Geometry check sheet. Reference: the model listing, model coordinates, mm. Face numbers are marked on the shaded views. A direction names the side the tool comes from. Round coordinates to 2 decimals unless told otherwise and drop trailing zeros. Write each loop counter-clockwise with the first axis right and the second up, starting at its lowest first coordinate (ties: lowest second). Pieces come first, ordered by that corner, then holes. Notation, with made-up numbers: (36.5, 31) - (69.5, 31) arc R22 ccw to (69.5, 39) - close; hole circle Ø2 at (43.25, -14.75). An arc over 180 degrees is marked (long way). Return JSON: item names as keys, results as strings. Group by question number.
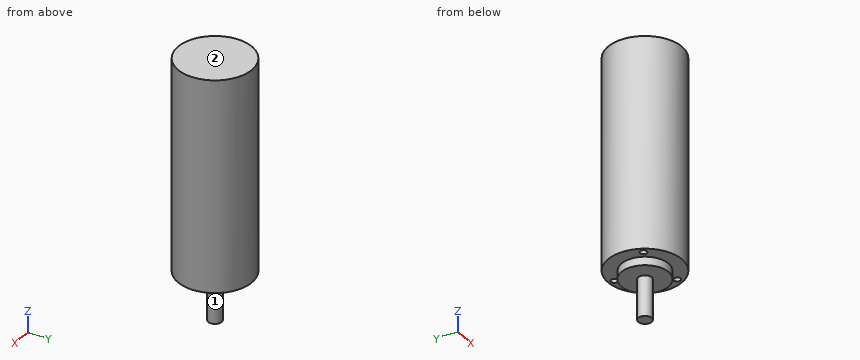
from build123d import *

# Parameters (mm, degrees)
SKETCH2_R          = 1
CUT_EXTRUDE1_DEPTH = 3


with BuildPart() as part:
    # Sketch1 → Revolve1 (revolve)
    with BuildSketch(Plane(origin=(0, 0, 0), x_dir=(1, 0, 0), z_dir=(0, 1, 0))):
        Polygon((0, 0), (11, 0), (11, 62.8), (7, 62.8), (7, 65.3), (2, 65.3), (2, 77.3), (0, 77.3), align=None)
    revolve(axis=Axis((0, 0, 0), (0, 0, -1)))

    # Sketch2 → Cut-Extrude1 (cut)
    with BuildSketch(Plane(origin=(0, 0, -62.8), x_dir=(-1, 0, 0), z_dir=(0, 0, -1))):
        with Locations((-8, -4.618802154)):
            Circle(SKETCH2_R)
        with Locations((0, 9.237604307)):
            Circle(SKETCH2_R)
        with Locations((8, -4.618802154)):
            Circle(SKETCH2_R)
    extrude(amount=-CUT_EXTRUDE1_DEPTH, mode=Mode.SUBTRACT)


solid = part.part
1. Section check C-C (y = 5). Enter the section's corners in (x, z), and give its area (3 significant figures).
2. Tool access check on the marked faces 1 and 2. Record the directions out of +Z, -Z, +X, -X, +Y, -Y that give a thin tool (end or side, any length) a straight path to the whole face; none if there is none.
3. Material ranges on line 1 along Z through (x, y) = (5, 8); line 2 along Y through (x, z) = (-8, -61.35); line 3 along Z through (x, y) = (-1.5, -2.5), recorded low to high.
4. Section check D-D (x = 4). Enter the section's corners in (y, z), and give its area (3 significant figures).
5. Section check B-B (z = -21). Enter the section's corners in (x, y).
6. Section check A-A (x = 0). Enter the section's corners in (y, z), and give its area (3 significant figures).
7. Depth check by flat-ended pin: pin 1 Ø1.5 at (x, z) = (-2.5, -35) entering from -Y; pin 2 Ø4 at (x, y) = (6, -1.5) entering from -Z; pin 3 Ø2 at (y, z) = (3.5, -24) entering from +X. Enter the tip coordinate at first touch or a pass-through.
Result sheet:
{
 "1": {"outline": "(-9.8, -62.8) - (-4.9, -62.8) - (-4.9, -65.3) - (4.9, -65.3) - (4.9, -62.8) - (9.8, -62.8) - (9.8, 0) - (-9.8, 0) - close", "area": "1,260 mm²"},
 "2": {"face 1": "-Z", "face 2": "+Z, +X, -X, +Y, -Y"},
 "3": {"line 1": "z = -62.8 to 0", "line 2": "y = -7.55 to -5.62, -3.62 to 7.55", "line 3": "z = -65.3 to 0"},
 "4": {"outline": "(-10.25, -62.8) - (-5.74, -62.8) - (-5.74, -65.3) - (5.74, -65.3) - (5.74, -62.8) - (10.25, -62.8) - (10.25, 0) - (-10.25, 0) - close", "area": "1,320 mm²"},
 "5": {"outline": "circle Ø22 at (0, 0)"},
 "6": {"outline": "(-11, -62.8) - (-7, -62.8) - (-7, -65.3) - (-2, -65.3) - (-2, -77.3) - (2, -77.3) - (2, -65.3) - (7, -65.3) - (7, -62.8) - (8.24, -62.8) - (8.24, -59.8) - (10.24, -59.8) - (10.24, -62.8) - (11, -62.8) - (11, 0) - (-11, 0) - close", "area": "1,460 mm²"},
 "7": {"pin 1": "stops at y = -10.86", "pin 2": "stops at z = -65.3", "pin 3": "stops at x = 10.71"}
}
